Can you work these out from the model? Positions are in its coordinate system, mm. A direction names the side the tool comes from. Give positions to 0.01 mm unless a question says otherwise; leave off trailing zeros. Write each loop counter-clockwise with the first axis right and the second up, starting at its lowest first coordinate (ties: lowest second). Pieces come first, ordered by that corner, then holes.
from build123d import *

# Parameters (mm, degrees)
SHELL1_T = -1


with BuildPart() as part:
    # Sketch1 → Revolve1 (revolve)
    with BuildSketch(Plane(origin=(0, 0, 0), x_dir=(1, 0, 0), z_dir=(0, 1, 0)), mode=Mode.PRIVATE) as revolve1_sk:
        Polygon((0, 9.75), (2.5, 9.75), (2.5, 3.75), (4, 3.75), (4, -7.75), (2.5, -7.75), (2.5, -9.75), (0, -9.75), align=None)
    revolve(revolve1_sk.sketch.rotate(Axis((0, 0, -28.532608696), (0, 0, 1)), 180), axis=Axis((0, 0, -28.532608696), (0, 0, 1)))

    # Shell1
    shell1_openings = [part.faces().sort_by_distance(p)[0] for p in [
        (0, 0, 9.75),
        (0, 0, -9.75),
    ]]
    offset(amount=SHELL1_T, openings=shell1_openings, kind=Kind.INTERSECTION)


solid = part.part
(1) Imagine slicing it at D-D, the plane y = -1.75. Write out the boundary of the cut face in (x, z).
Returned:
outline: (-3.6, -3.75) - (-1.79, -3.75) - (-1.79, -9.75) - (1.79, -9.75) - (1.79, -3.75) - (3.6, -3.75) - (3.6, 7.75) - (1.79, 7.75) - (1.79, 9.75) - (-1.79, 9.75) - (-1.79, 7.75) - (-3.6, 7.75) - close; hole (-2.44, -2.75) - (2.44, -2.75) - (2.44, 6.75) - (-2.44, 6.75) - close
(2) For faces 4 (the face through (2, -2, -3.75)), 5 (the face through (-2.86, -0.9, 2.07)), 6 (the face through (2.5, -0.1, 8.8)), which set-ups out of +Z, -Z, +X, -X, +Y, -Y let a thin tool reach every point of the face, with its end or its side?
Returned:
face 4: -Z
face 5: none
face 6: +Z
(3) Imagine slicing it at A-A, the plane x = 0. Write out the boundary of the cut face in (y, z).
Returned:
outline: (-4, -3.75) - (-2.5, -3.75) - (-2.5, -9.75) - (-1.5, -9.75) - (-1.5, -2.75) - (-3, -2.75) - (-3, 6.75) - (-1.5, 6.75) - (-1.5, 9.75) - (-2.5, 9.75) - (-2.5, 7.75) - (-4, 7.75) - close; (1.5, -9.75) - (2.5, -9.75) - (2.5, -3.75) - (4, -3.75) - (4, 7.75) - (2.5, 7.75) - (2.5, 9.75) - (1.5, 9.75) - (1.5, 6.75) - (3, 6.75) - (3, -2.75) - (1.5, -2.75) - close
(4) Imagine slicing it at C-C, the plane z = 6. Write out the boundary of the cut face in (x, y), plus the area to 3 significant figures.
Returned:
outline: circle Ø8 at (0, 0); hole circle Ø6 at (0, 0)
area: 22.0 mm2
(5) If we mould it in two halves opening along Y, with no side actions, what happens to faces 1 (the face through (1.3, 1.3, -2.75)), 2 (the face through (-2, -2, 7.75)), 3 (the face through (2.5, -0.1, -6.7))? For each: +Y half, -Y half, draft (parallel to the pull), parting line (faces both ways), or undercut.
Returned:
face 1: undercut
face 2: draft
face 3: parting line
(6) Will these pins go through, and if not, where does the flat tip stop? P1, Ø1.8, axis at x = 0, y = 0, coming from the -Z side; P2, Ø4, axis at y = -2.5, z = 7, coming from the +X side.
Returned:
P1: passes through
P2: stops at x = 3.97
(7) If I drill on L1, parallel to Y at x = 0, z = 7.85; L2, parallel to Z at x = 0.5, y = 2.5; L3, parallel to Z at x = -1.5, y = 0.5, over which ranges is the centre line in solid material (lowest first)?
Returned:
L1: y = -2.5 to -1.5, 1.5 to 2.5
L2: z = -3.75 to -2.75, 6.75 to 7.75
L3: z = -9.75 to -2.75, 6.75 to 9.75
